from build123d import *

# Parameters (mm, degrees)
SKETCH1_R               = 3.175
SKETCH1_R_2             = 3.1115
BOSS_EXTRUDE1_DEPTH     = 50.8
CUT_EXTRUDE1_DEPTH      = 3.81
CUT_EXTRUDE6_DEPTH      = 94.132822302
CUT_EXTRUDE7_DEPTH      = 81.280992342
CUT_EXTRUDE7_DEPTH_BACK = 81.280992342
SKETCH8_W               = 18.542
SKETCH8_H               = 31.75
SKETCH9_R               = 3.429
SKETCH9_R_2             = 3.3655
CUT_EXTRUDE8_DEPTH      = 77.458810064
FILLET1_R               = 2.54


with BuildPart() as part:
    # Sketch1 → Boss-Extrude1 (new body)
    with BuildSketch(Plane.XY):
        Polygon((-3.17337999, 28.220199493), (-67.093802786, -13.260151874), (-49.810323049, -39.893661373), (14.110099747, 1.586689995), align=None)
        Circle(SKETCH1_R, mode=Mode.SUBTRACT)
        with Locations((-42.613615197, -27.653567579)):
            Circle(SKETCH1_R, mode=Mode.SUBTRACT)
        with Locations((-21.306807599, -13.826783789)):
            Circle(SKETCH1_R_2, mode=Mode.SUBTRACT)
    extrude(amount=-BOSS_EXTRUDE1_DEPTH)

    # Sketch2 → Cut-Extrude1 (cut, symmetric)
    with BuildSketch(Plane.XY.offset(-25.4)):
        Polygon((-36.108246535, -14.348133404), (-57.415054133, -28.174917194), (-49.810323049, -39.893661373), (-39.15691925, -32.980269478), (-28.503515451, -26.066877584), align=None)
        Polygon((-14.801438936, -0.521349615), (6.505368663, 13.305434174), (14.110099747, 1.586689995), (3.456695947, -5.3267019), (-7.196707852, -12.240093794), align=None)
    extrude(amount=CUT_EXTRUDE1_DEPTH, both=True, mode=Mode.SUBTRACT)

    # Sketch7 → Cut-Extrude6 (cut, through all)
    with BuildSketch(Plane.XY):
        with BuildLine():
            Line((-47.65700114, -8.216765932), (-37.286913298, -24.196871631))
            ThreePointArc((-37.286913298, -24.196871631), (-36.524811659, -25.851077227), (-36.263615197, -27.653567579))
            ThreePointArc((-36.263615197, -27.653567579), (-37.033627746, -30.684448646), (-39.156919149, -32.980269413))
            Line((-39.156919149, -32.980269413), (-17.850111759, -19.153485759))
            ThreePointArc((-17.850111759, -19.153485759), (-22.629101551, -20.037583955), (-26.633509498, -17.283479737))
            Line((-26.633509498, -17.283479737), (-37.00359734, -1.303374038))
            Line((-37.00359734, -1.303374038), (-47.65700114, -8.216765932))
        make_face()
        with BuildLine():
            ThreePointArc((-14.956807599, -13.826783789), (-15.726820207, -16.857664966), (-17.850111759, -19.153485759))
            Line((-17.850111759, -19.153485759), (3.456695863, -5.326701954))
            ThreePointArc((3.456695863, -5.326701954), (-1.322293939, -6.210800169), (-5.3267019, -3.456695947))
            Line((-5.3267019, -3.456695947), (-15.696789742, 12.523409752))
            Line((-15.696789742, 12.523409752), (-26.350193541, 5.610017857))
            Line((-26.350193541, 5.610017857), (-15.980105699, -10.370087842))
            ThreePointArc((-15.980105699, -10.370087842), (-15.21800406, -12.024293437), (-14.956807599, -13.826783789))
        make_face()
        with BuildLine():
            ThreePointArc((6.35, 0), (5.579987398, -3.030881165), (3.456695863, -5.326701954))
            Line((3.456695863, -5.326701954), (14.110099747, 1.586689995))
            Line((14.110099747, 1.586689995), (0.283315957, 22.893497594))
            Line((0.283315957, 22.893497594), (6.122209073, 1.685543256))
            ThreePointArc((6.122209073, 1.685543256), (6.292794594, 0.850432945), (6.35, 0))
        make_face()
        with BuildLine():
            ThreePointArc((-39.156919149, -32.980269413), (-42.970845505, -33.993511309), (-46.646808241, -32.558244313))
            Line((-46.646808241, -32.558244313), (-63.637106839, -18.586853774))
            Line((-63.637106839, -18.586853774), (-49.810323049, -39.893661373))
            Line((-49.810323049, -39.893661373), (-39.156919149, -32.980269413))
        make_face()
    extrude(amount=-CUT_EXTRUDE6_DEPTH, mode=Mode.SUBTRACT)

    # Sketch8 → Cut-Extrude7 (cut, two sides: drawn at the far end of the back side and taken through both)
    with BuildSketch(Plane(origin=(-21.306807599, -13.826783789, 0), x_dir=(0, 0, -1), z_dir=(0.838850692859666, 0.5443615665059929, 0)).offset(-CUT_EXTRUDE7_DEPTH_BACK)):
        with Locations((9.271, 9.525)):
            Rectangle(SKETCH8_W, SKETCH8_H)
        with Locations((41.529, 9.525)):
            Rectangle(SKETCH8_W, SKETCH8_H)
    extrude(amount=CUT_EXTRUDE7_DEPTH + CUT_EXTRUDE7_DEPTH_BACK, mode=Mode.SUBTRACT)

    # Sketch9 → Cut-Extrude8 (cut, through all)
    with BuildSketch(Plane(origin=(0, 0, -32.258), x_dir=(-1, 0, 0), z_dir=(0, 0, -1))):
        Circle(SKETCH9_R)
        with Locations((21.306807599, -13.826783789)):
            Circle(SKETCH9_R_2)
        with Locations((42.613615197, -27.653567579)):
            Circle(SKETCH9_R)
    extrude(amount=-CUT_EXTRUDE8_DEPTH, mode=Mode.SUBTRACT)

    # Fillet1
    fillet1_edges = [part.edges().sort_by_distance(p)[0] for p in [
        (-15.696789742, 12.523409752, -25.4),
        (-26.350193541, 5.610017857, -25.4),
        (-37.00359734, -1.303374038, -25.4),
        (-47.65700114, -8.216765932, -25.4),
    ]]
    fillet(fillet1_edges, radius=FILLET1_R)


solid = part.part
The listing builds one solid part. Answer for the finished solid, in the listing's coordinates (mm). A direction names the side the tool comes from. Round coordinates to 2 decimals unless told otherwise and drop trailing zeros. Write each loop counter-clockwise with the first axis right and the second up, starting at its lowest first coordinate (ties: lowest second). Pieces come first, ordered by that corner, then holes. Notation, with made-up numbers: (63.25, 57) - (89.25, 57) arc R33 cw to (89.25, 89) - close; hole circle Ø6 at (3.5, 0.5). An arc over 180 degrees is marked (long way). Use a Markdown table: item, result. Add a question column.
1. The part is cut by section A-A (z = -23). Write down the section's boundary in (x, y), and give its area (3 significant figures).
2. Flat-ended cylindrical pins translate along their axes: P1, Ø1, axis at x = -36.5, z = -28.5, coming from the +Y side; P2, Ø2, axis at x = -43.5, z = -25, coming from the +Y side; P3, Ø8, axis at y = 5.5, z = -21.5, coming from the +X side. Find the tip coordinate at first contact, or state that the pin passes through.
3. A tool of negligible diameter and unlimited length cuts with its end or side. For faces 1 (the face through (-56.91, -24.12, -25.3)), 2 (the face through (-31.06, -10.46, -25.3)), 3 (the face through (-3, 3, -29.21)), 4 (the face through (-31, 0, -32.258)), 5 (the face through (-15.89, 11.49, -25.5)), from which of +Z, -Z, +X, -X, +Y, -Y can it reach the whole face along a straight path? Write none if from no direction.
4. The part is cut by section B-B (y = 8). Write down the section's boundary in (x, z), and give its area (3 significant figures).
5. Consider line 1 (X direction, y = -14, z = -25.25); line 2 (Y direction, x = -41, z = -21); line 3 (X direction, y = -3, z = -19.5). Determine where each line is inside the solid, lowest interval first.
6. For a pull along X with two mould halves and no side action, classify faces 6 (the face through (-1.42, 25.52, -25.3)), 7 (the face through (-42.84, -15.64, -25.3)), 8 (the face through (-34.69, 7.77, -25.3)) as +X half, -X half, draft (parallel to the pull), parting line (faces both ways), or undercut.
7. The part is cut by section C-C (z = -30.5). Write down the section's boundary in (x, y).
8. The part is cut by section D-D (y = -8). Write down the section's boundary in (x, z).
Reported:
| question | item | result |
|---|---|---|
| 1 | outline | (-67.09, -13.26) - (-63.64, -18.59) - (-54.38, -26.2) - (-41.43, -17.8) - (-46.27, -10.35) arc R2.54 cw to (-45.53, -6.83) - (-39.13, -2.69) arc R2.54 cw to (-35.62, -3.43) - (-26.63, -17.28) arc R6.35 ccw to (-15.98, -10.37) - (-24.97, 3.48) arc R2.54 cw to (-24.22, 6.99) - (-17.83, 11.14) arc R2.54 cw to (-14.31, 10.39) - (-9.47, 2.94) - (3.47, 11.33) - (0.28, 22.89) - (-3.17, 28.22) - close; hole circle Ø6.73 at (-21.31, -13.83) |
| 1 | area | 1,150 mm^2 |
| 2 | P1 | y = 6.92 |
| 2 | P2 | y = 2.7 |
| 2 | P3 | x = 6.17 |
| 3 | face 1 | +Z, -Z, -X, -Y |
| 3 | face 2 | +Z, -Z, -Y |
| 3 | face 3 | +X, -Y |
| 3 | face 4 | -Z, +X, -X, +Y, -Y |
| 3 | face 5 | +Z, -Z |
| 4 | outline | (-34.33, -32.26) - (-22.67, -32.26) - (-22.67, -18.54) - (-34.33, -18.54) - close; (-12.76, -32.26) - (4.38, -32.26) - (4.38, -29.21) - (-1.67, -29.21) - (-1.67, -21.59) - (4.38, -21.59) - (4.38, -18.54) - (-12.76, -18.54) - close |
| 4 | area | 349 mm^2 |
| 5 | line 1 | -66.61 to -43.9, -28.76 to -24.67, -17.95 to -14.96 |
| 5 | line 2 | -33.8 to -30.68, -24.63 to -18.48, -3.9 to 3.67 |
| 5 | line 3 | -51.28 to -39.62, -35.98 to -20.76, -5.62 to -1.66, 1.66 to 5.6 |
| 6 | face 6 | +X half |
| 6 | face 7 | undercut |
| 6 | face 8 | -X half |
| 7 | outline | (-67.09, -13.26) - (-63.64, -18.59) - (-46.65, -32.56) arc R6.35 ccw to (-37.29, -24.2) - (-46.27, -10.35) arc R2.54 cw to (-45.53, -6.83) - (-39.13, -2.69) arc R2.54 cw to (-35.62, -3.43) - (-26.63, -17.28) arc R6.35 ccw to (-15.98, -10.37) - (-24.97, 3.48) arc R2.54 cw to (-24.22, 6.99) - (-17.83, 11.14) arc R2.54 cw to (-14.31, 10.39) - (-5.33, -3.46) arc R6.35 ccw to (6.12, 1.69) - (0.28, 22.89) - (-3.17, 28.22) - close; hole circle Ø6.86 at (-42.61, -27.65); hole circle Ø6.73 at (-21.31, -13.83); hole circle Ø6.86 at (0, 0) |
| 8 | outline | (-58.99, -32.26) - (-46.49, -32.26) - (-46.49, -18.54) - (-58.99, -18.54) - close; (-32.66, -32.26) - (-17.52, -32.26) - (-17.52, -18.54) - (-32.66, -18.54) - close |
